from build123d import *

# Parameters (mm, degrees)
SKETCH1_R           = 17
SKETCH1_R_2         = 15.796210214
SKETCH1_R_3         = 14.369088414
SKETCH1_R_4         = 13.369088414
SKETCH1_R_5         = 10.562338101
SKETCH1_R_6         = 9.108597541
SKETCH1_R_7         = 7.390019335
SKETCH1_R_8         = 5.587157692
BOSS_EXTRUDE1_DEPTH = 2
SKETCH1_3_R         = 14.369088414
SKETCH1_3_R_2       = 13.369088414
SKETCH1_3_R_3       = 10.562338101
SKETCH1_3_R_4       = 9.108597541
SKETCH1_3_R_5       = 7.390019335
SKETCH1_3_R_6       = 5.587157692
BOSS_EXTRUDE2_DEPTH = 10
CHAMFER3_SIZE       = 5
CHAMFER4_SIZE       = 0.5
CHAMFER5_SIZE       = 0.5


with BuildPart() as part:
    # Sketch1 → Boss-Extrude1 (new body)
    # profile 1 of 8: a face of its own
    with BuildSketch(Plane.XY):
        Circle(SKETCH1_R)
        Circle(SKETCH1_R_2, mode=Mode.SUBTRACT)
    # profile 2 of 8: a face of its own
    with BuildSketch(Plane.XY):
        Circle(SKETCH1_R_2)
        Circle(SKETCH1_R_3, mode=Mode.SUBTRACT)
    # profile 3 of 8: a face of its own
    with BuildSketch(Plane.XY):
        Circle(SKETCH1_R_3)
        Circle(SKETCH1_R_4, mode=Mode.SUBTRACT)
    # profile 4 of 8: a face of its own
    with BuildSketch(Plane.XY):
        Circle(SKETCH1_R_4)
        Circle(SKETCH1_R_5, mode=Mode.SUBTRACT)
    # profile 5 of 8: a face of its own
    with BuildSketch(Plane.XY):
        Circle(SKETCH1_R_5)
        Circle(SKETCH1_R_6, mode=Mode.SUBTRACT)
    # profile 6 of 8: a face of its own
    with BuildSketch(Plane.XY):
        Circle(SKETCH1_R_6)
        Circle(SKETCH1_R_7, mode=Mode.SUBTRACT)
    # profile 7 of 8: a face of its own
    with BuildSketch(Plane.XY):
        Circle(SKETCH1_R_7)
        Circle(SKETCH1_R_8, mode=Mode.SUBTRACT)
    # profile 8 of 8: a face of its own
    with BuildSketch(Plane.XY):
        Circle(SKETCH1_R_8)
    extrude(amount=-BOSS_EXTRUDE1_DEPTH)

    # Sketch1<3> → Boss-Extrude2 (add)
    # profile 1 of 3: a face of its own
    with BuildSketch(Plane.XY):
        Circle(SKETCH1_3_R)
        Circle(SKETCH1_3_R_2, mode=Mode.SUBTRACT)
    # profile 2 of 3: a face of its own
    with BuildSketch(Plane.XY):
        Circle(SKETCH1_3_R_3)
        Circle(SKETCH1_3_R_4, mode=Mode.SUBTRACT)
    # profile 3 of 3: a face of its own
    with BuildSketch(Plane.XY):
        Circle(SKETCH1_3_R_5)
        Circle(SKETCH1_3_R_6, mode=Mode.SUBTRACT)
    extrude(amount=BOSS_EXTRUDE2_DEPTH)

    # Chamfer3
    chamfer3_edges = [part.edges().sort_by_distance(p)[0] for p in [
        (-5.587157692, 0, 0),
    ]]
    chamfer(chamfer3_edges, length=CHAMFER3_SIZE)

    # Chamfer4
    chamfer4_edges = [part.edges().sort_by_distance(p)[0] for p in [
        (-9.108597541, 0, 0),
        (-10.562338101, 0, 0),
        (-7.390019335, 0, 0),
        (-14.369088414, 0, 0),
        (-13.369088414, 0, 0),
    ]]
    chamfer(chamfer4_edges, length=CHAMFER4_SIZE)

    # Chamfer5
    chamfer5_edges = [part.edges().sort_by_distance(p)[0] for p in [
        (-9.108597541, 0, 10),
        (-10.562338101, 0, 10),
        (-5.587157692, 0, 10),
        (-7.390019335, 0, 10),
        (-13.369088414, 0, 10),
        (-14.369088414, 0, 10),
    ]]
    chamfer(chamfer5_edges, length=CHAMFER5_SIZE - 0.0001)  # a hair under: the kernel refuses the full size


solid = part.part
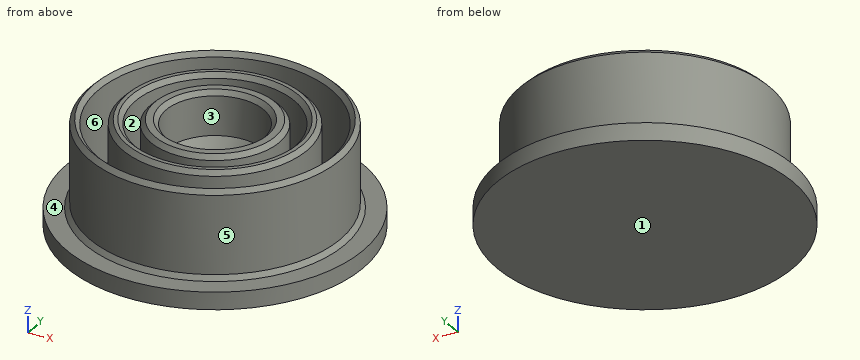
Verification items for the finished model (mm, model axes). Face numbers are marked on the shaded views. A direction names the side the tool comes from. Give positions to 0.01 mm unless a question says otherwise; leave off trailing zeros. Write each loop counter-clockwise with the first axis right and the second up, starting at its lowest first coordinate (ties: lowest second). Pieces come first, ordered by that corner, then holes.
(1) Cross-section at B-B (z = 4.5). Enter the section's corners in (x, y), plus the area to 3 significant figures.
(2) Mould release check, pull along X, two halves, no side actions. Record for the marked faces 3, 4, 5 and 6: +X half, -X half, draft (parallel to the pull), parting line (faces both ways), or undercut.
(3) Material ranges on line 1 (Y direction, x = 0, z = 6.3); line 2 (X direction, y = -4, z = 0.75); line 3 (Y direction, x = 5, z = 3.5), recorded low to high.
(4) Cross-section at A-A (z = 6.25). Enter the section's corners in (x, y), plus the area to 3 significant figures.
(5) Gauge pin test, flat ends, axial feed: pin 1 (1 mm diameter, centred on y = 11, z = 7, fed in from -X); pin 2 (1.5 mm diameter, centred on y = 7, z = 0, fed in from +X); pin 3 (5 mm diameter, centred on x = -1.5, z = 5.5, fed in from +Y). Record the tip position at first contact, or that the pin passes through.
(6) Cross-section at C-C (y = 15.5). Enter the section's corners in (x, z).
(7) Access from +Z, -Z, +X, -X, +Y, -Y to the whole of each face (thin tool, end or side, straight path). Record for the marked faces 1 and 2.
Worked out:
1. outline: circle Ø28.74 at (0, 0); circle Ø21.12 at (0, 0); circle Ø14.78 at (0, 0); hole circle Ø26.74 at (0, 0); hole circle Ø18.22 at (0, 0); hole circle Ø10.17 at (0, 0)
1. area: 267 mm2
2. face 3: undercut
2. face 4: draft
2. face 5: parting line
2. face 6: undercut
3. line 1: y = -14.37 to -13.37, -10.56 to -9.11, -7.39 to -5.59, 5.59 to 7.39, 9.11 to 10.56, 13.37 to 14.37
3. line 2: x = -13.8 to -12.76, -9.78 to -8.18, -6.21 to 6.21, 8.18 to 9.78, 12.76 to 13.8
3. line 3: y = -13.47 to -12.4, -9.3 to -7.61, -5.44 to 5.44, 7.61 to 9.3, 12.4 to 13.47
4. outline: circle Ø28.74 at (0, 0); circle Ø21.12 at (0, 0); circle Ø14.78 at (0, 0); hole circle Ø26.74 at (0, 0); hole circle Ø18.22 at (0, 0); hole circle Ø11.17 at (0, 0)
4. area: 250 mm2
5. pin 1: stops at x = -9.81
5. pin 2: stops at x = 15.81
5. pin 3: stops at y = 14.37
6. outline: (-6.98, -2) - (6.98, -2) - (6.98, 0) - (-6.98, 0) - close
7. face 1: -Z, +X, -X, +Y, -Y
7. face 2: +Z
